```python
from build123d import *

# Parameters (mm, degrees)
PAD_DEPTH        = 1
POCKET_DEPTH     = 0.001
HOLE_D           = 1.75
HOLE_CSINK_D     = 3.3
HOLE_CSINK_ANGLE = 90
SKETCH025_R      = 5.25
SKETCH025_R_2    = 1.5
POCKET007_DEPTH  = 5
POCKET008_DEPTH  = 1.001


with BuildPart() as part:
    # Sketch → Pad (new body)
    with BuildSketch(Plane.XY):
        with BuildLine():
            Line((-51.8, 52.175), (51.8, 52.175))
            ThreePointArc((52.175, 51.8), (52.065165, 52.065165), (51.8, 52.175))
            Line((52.175, 51.8), (52.175, -51.8))
            ThreePointArc((51.8, -52.175), (52.065165, -52.065165), (52.175, -51.8))
            Line((51.8, -52.175), (-51.8, -52.175))
            ThreePointArc((-52.175, -51.8), (-52.065165, -52.065165), (-51.8, -52.175))
            Line((-52.175, -51.8), (-52.175, 51.8))
            ThreePointArc((-51.8, 52.175), (-52.065165, 52.065165), (-52.175, 51.8))
        make_face()
    extrude(amount=-PAD_DEPTH)

    # Sketch002 → Pocket (cut, through all)
    with BuildSketch(Plane.XY.offset(-4.8)):
        with BuildLine():
            Line((-45, 50.175), (45, 50.175))
            ThreePointArc((45, 50.175), (45.353553, 50.321447), (45.5, 50.675))
            ThreePointArc((45.5, 50.675), (45.353553, 51.028553), (45, 51.175))
            Line((-45, 51.175), (45, 51.175))
            ThreePointArc((-45, 51.175), (-45.353553, 51.028553), (-45.5, 50.675))
            ThreePointArc((-45.5, 50.675), (-45.353553, 50.321447), (-45, 50.175))
        make_face()
        with BuildLine():
            Line((-45, -51.175), (45, -51.175))
            ThreePointArc((45, -51.175), (45.353553, -51.028553), (45.5, -50.675))
            ThreePointArc((45.5, -50.675), (45.353553, -50.321447), (45, -50.175))
            Line((-45, -50.175), (45, -50.175))
            ThreePointArc((-45, -50.175), (-45.353553, -50.321447), (-45.5, -50.675))
            ThreePointArc((-45.5, -50.675), (-45.353553, -51.028553), (-45, -51.175))
        make_face()
        with BuildLine():
            Line((51.175, -45), (51.175, 45))
            ThreePointArc((51.175, 45), (51.028553, 45.353553), (50.675, 45.5))
            ThreePointArc((50.675, 45.5), (50.321447, 45.353553), (50.175, 45))
            Line((50.175, -45), (50.175, 45))
            ThreePointArc((50.175, -45), (50.321447, -45.353553), (50.675, -45.5))
            ThreePointArc((50.675, -45.5), (51.028553, -45.353553), (51.175, -45))
        make_face()
        with BuildLine():
            Line((-50.175, -45), (-50.175, 45))
            ThreePointArc((-50.175, 45), (-50.321447, 45.353553), (-50.675, 45.5))
            ThreePointArc((-50.675, 45.5), (-51.028553, 45.353553), (-51.175, 45))
            Line((-51.175, -45), (-51.175, 45))
            ThreePointArc((-51.175, -45), (-51.028553, -45.353553), (-50.675, -45.5))
            ThreePointArc((-50.675, -45.5), (-50.321447, -45.353553), (-50.175, -45))
        make_face()
    extrude(amount=-POCKET_DEPTH, mode=Mode.SUBTRACT)

    # Hole (through all)
    with Locations(Plane.XY):
        with Locations((-50, 50), (50, 50), (50, -50), (-50, -50)):
            CounterSinkHole(HOLE_D / 2, HOLE_CSINK_D / 2, counter_sink_angle=HOLE_CSINK_ANGLE)

    # Sketch025 → Pocket007 (cut)
    with BuildSketch(Plane.XY):
        with Locations((-26.67, 26.67)):
            Circle(SKETCH025_R)
        with Locations((26.67, 26.67)):
            Circle(SKETCH025_R)
        with Locations((-47.515079, 36.39022)):
            Circle(SKETCH025_R_2)
        with Locations((-45.510497, 39.862258)):
            Circle(SKETCH025_R_2)
        with Locations((-42.933456, 42.933456)):
            Circle(SKETCH025_R_2)
        with Locations((-39.862258, 45.510497)):
            Circle(SKETCH025_R_2)
        with Locations((-36.39022, 47.515079)):
            Circle(SKETCH025_R_2)
        with Locations((5.824921, 36.39022)):
            Circle(SKETCH025_R_2)
        with Locations((7.829503, 39.862258)):
            Circle(SKETCH025_R_2)
        with Locations((10.406544, 42.933456)):
            Circle(SKETCH025_R_2)
        with Locations((13.477742, 45.510497)):
            Circle(SKETCH025_R_2)
        with Locations((16.94978, 47.515079)):
            Circle(SKETCH025_R_2)
    extrude(amount=-POCKET007_DEPTH, mode=Mode.SUBTRACT)

    # Sketch023 → Pocket008 (cut, through all)
    with BuildSketch(Plane.XY):
        with BuildLine():
            Line((-48.505, -19.735), (-48.505, -6.935))
            ThreePointArc((-46.405, -4.835), (-47.889924, -5.450076), (-48.505, -6.935))
            Line((-46.405, -4.835), (-33.605, -4.835))
            ThreePointArc((-31.505, -6.935), (-32.120076, -5.450076), (-33.605, -4.835))
            Line((-31.505, -6.935), (-31.505, -19.735))
            ThreePointArc((-33.605, -21.835), (-32.120076, -21.219924), (-31.505, -19.735))
            Line((-33.605, -21.835), (-46.405, -21.835))
            ThreePointArc((-48.505, -19.735), (-47.889924, -21.219924), (-46.405, -21.835))
        make_face()
        with BuildLine():
            Line((-21.835, -19.735), (-21.835, -6.935))
            ThreePointArc((-19.735, -4.835), (-21.219924, -5.450076), (-21.835, -6.935))
            Line((-19.735, -4.835), (-6.935, -4.835))
            ThreePointArc((-4.835, -6.935), (-5.450076, -5.450076), (-6.935, -4.835))
            Line((-4.835, -6.935), (-4.835, -19.735))
            ThreePointArc((-6.935, -21.835), (-5.450076, -21.219924), (-4.835, -19.735))
            Line((-6.935, -21.835), (-19.735, -21.835))
            ThreePointArc((-21.835, -19.735), (-21.219924, -21.219924), (-19.735, -21.835))
        make_face()
        with BuildLine():
            Line((4.835, -19.735), (4.835, -6.935))
            ThreePointArc((6.935, -4.835), (5.450076, -5.450076), (4.835, -6.935))
            Line((6.935, -4.835), (19.735, -4.835))
            ThreePointArc((21.835, -6.935), (21.219924, -5.450076), (19.735, -4.835))
            Line((21.835, -6.935), (21.835, -19.735))
            ThreePointArc((19.735, -21.835), (21.219924, -21.219924), (21.835, -19.735))
            Line((19.735, -21.835), (6.935, -21.835))
            ThreePointArc((4.835, -19.735), (5.450076, -21.219924), (6.935, -21.835))
        make_face()
        with BuildLine():
            Line((31.505, -19.735), (31.505, -6.935))
            ThreePointArc((33.605, -4.835), (32.120076, -5.450076), (31.505, -6.935))
            Line((33.605, -4.835), (46.405, -4.835))
            ThreePointArc((48.505, -6.935), (47.889924, -5.450076), (46.405, -4.835))
            Line((48.505, -6.935), (48.505, -19.735))
            ThreePointArc((46.405, -21.835), (47.889924, -21.219924), (48.505, -19.735))
            Line((46.405, -21.835), (33.605, -21.835))
            ThreePointArc((31.505, -19.735), (32.120076, -21.219924), (33.605, -21.835))
        make_face()
        with BuildLine():
            Line((31.505, -46.405), (31.505, -33.605))
            ThreePointArc((33.605, -31.505), (32.120076, -32.120076), (31.505, -33.605))
            Line((33.605, -31.505), (46.405, -31.505))
            ThreePointArc((48.505, -33.605), (47.889924, -32.120076), (46.405, -31.505))
            Line((48.505, -33.605), (48.505, -46.405))
            ThreePointArc((46.405, -48.505), (47.889924, -47.889924), (48.505, -46.405))
            Line((46.405, -48.505), (33.605, -48.505))
            ThreePointArc((31.505, -46.405), (32.120076, -47.889924), (33.605, -48.505))
        make_face()
        with BuildLine():
            Line((4.835, -46.405), (4.835, -33.605))
            ThreePointArc((6.935, -31.505), (5.450076, -32.120076), (4.835, -33.605))
            Line((6.935, -31.505), (19.735, -31.505))
            ThreePointArc((21.835, -33.605), (21.219924, -32.120076), (19.735, -31.505))
            Line((21.835, -33.605), (21.835, -46.405))
            ThreePointArc((19.735, -48.505), (21.219924, -47.889924), (21.835, -46.405))
            Line((19.735, -48.505), (6.935, -48.505))
            ThreePointArc((4.835, -46.405), (5.450076, -47.889924), (6.935, -48.505))
        make_face()
        with BuildLine():
            Line((-21.835, -46.405), (-21.835, -33.605))
            ThreePointArc((-19.735, -31.505), (-21.219924, -32.120076), (-21.835, -33.605))
            Line((-19.735, -31.505), (-6.935, -31.505))
            ThreePointArc((-4.835, -33.605), (-5.450076, -32.120076), (-6.935, -31.505))
            Line((-4.835, -33.605), (-4.835, -46.405))
            ThreePointArc((-6.935, -48.505), (-5.450076, -47.889924), (-4.835, -46.405))
            Line((-6.935, -48.505), (-19.735, -48.505))
            ThreePointArc((-21.835, -46.405), (-21.219924, -47.889924), (-19.735, -48.505))
        make_face()
        with BuildLine():
            Line((-48.505, -46.405), (-48.505, -33.605))
            ThreePointArc((-46.405, -31.505), (-47.889924, -32.120076), (-48.505, -33.605))
            Line((-46.405, -31.505), (-33.605, -31.505))
            ThreePointArc((-31.505, -33.605), (-32.120076, -32.120076), (-33.605, -31.505))
            Line((-31.505, -33.605), (-31.505, -46.405))
            ThreePointArc((-33.605, -48.505), (-32.120076, -47.889924), (-31.505, -46.405))
            Line((-33.605, -48.505), (-46.405, -48.505))
            ThreePointArc((-48.505, -46.405), (-47.889924, -47.889924), (-46.405, -48.505))
        make_face()
    extrude(amount=-POCKET008_DEPTH, mode=Mode.SUBTRACT)


solid = part.part
```
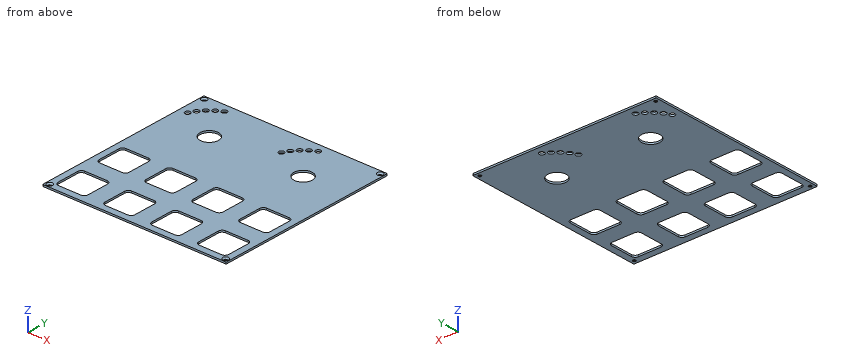
Input: part model. Units: mm. Frame: model coordinates. Round coordinates to 2 decimals unless told otherwise and drop trailing zeros. Order: outer loops, then holes, each group sorted by start corner. A loop starts at its lowest first (then second) coordinate and runs counter-clockwise, first axis right, second up. Notation, with made-up numbers: (30.5, 74) - (46.5, 74) arc R13 ccw to (46.5, 80) - close; hole circle Ø4 at (-17.75, -37.75). An arc over 180 degrees is marked (long way). One line per question, with ' | ' between items. Start each with the question number.
1) Cut plane C-C, the plane y = 26.67. Return the cut outline in (x, z) (3 decimals).
2) Contact query for a flat-ended pin moving along its axis: P1, Ø2.5, axis at x = -45.51, y = 39.86, coming from the -Z side. Output: stop coordinate, or through.
3) Cut plane D-D, the plane z = -0.4. Give the number of separate pieces and of enclosed holes in the cut face, then the cut area to 3 significant figures.
4) Cut plane B-B, the plane x = 26.67. Return the cut outline in (y, z) (3 decimals), then the cut area to 4 significant figures.
5) Cut plane A-A, the plane y = -16. Return the cut outline in (x, z) (3 decimals), then the cut area to 4 significant figures.
6) Ray query, probe 1 along X at (y, z) = (-10, -0.25) (3 decimals); probe 2 along X at (y, z) = (50, -0.9) (3 decimals); probe 3 along Y at (x, z) = (-36.5, -0.15) (3 decimals). Return the intervals inside material, ascending.
Worked out:
1) outline: (-52.175, -1) - (-31.92, -1) - (-31.92, 0) - (-52.175, 0) - close; (-21.42, -1) - (21.42, -1) - (21.42, 0) - (-21.42, 0) - close; (31.92, -1) - (52.175, -1) - (52.175, 0) - (31.92, 0) - close
2) P1: passes through
3) separate pieces: 1 | enclosed holes: 24 | area: 8,340 mm^2
4) outline: (-52.175, -1) - (21.42, -1) - (21.42, 0) - (-52.175, 0) - close; (31.92, -1) - (52.175, -1) - (52.175, 0) - (31.92, 0) - close | area: 93.85 mm^2
5) outline: (-52.175, -1) - (-48.505, -1) - (-48.505, 0) - (-52.175, 0) - close; (-31.505, -1) - (-21.835, -1) - (-21.835, 0) - (-31.505, 0) - close; (-4.835, -1) - (4.835, -1) - (4.835, 0) - (-4.835, 0) - close; (21.835, -1) - (31.505, -1) - (31.505, 0) - (21.835, 0) - close; (48.505, -1) - (52.175, -1) - (52.175, 0) - (48.505, 0) - close | area: 36.35 mm^2
6) probe 1: x = -52.175 to -48.505, -31.505 to -21.835, -4.835 to 4.835, 21.835 to 31.505, 48.505 to 52.175 | probe 2: x = -52.175 to -50.875, -49.125 to 49.125, 50.875 to 52.175 | probe 3: y = -52.175 to -48.505, -31.505 to -21.835, -4.835 to 46.019, 49.011 to 52.175
